Input: part model. Units: mm. Frame: model coordinates. A direction names the side the tool comes from. Give positions to 0.01 mm unless a question says otherwise; leave off trailing zeros. Loops run counter-clockwise (first coordinate to the right, second up) from the corner with the lowest first, then second, coordinate; pieces in that order, holes last. Notation, with made-up numbers: (-36, 64.25) -> (-22, 64.25) arc R25 ccw to (-22, 85.25) -> close; hole circle Ø7 at (-11.5, -5.75). An arc over 180 degrees is marked (long way). Answer as a JSON object with one key per item and string values.
```python
from build123d import *

# Parameters (mm, degrees)
F0_R     = 1.651
F1_DEPTH = 0.8128


with BuildPart() as f1:
    # F0 (on Front) → F1 (new body)
    with BuildSketch(Plane.XZ):
        with BuildLine():
            Line((-6.35, 36.576), (-8.89, 36.576))
            ThreePointArc((-8.89, 36.576), (-11.584077, 35.460077), (-12.7, 32.766))
            Line((-12.7, 32.766), (-12.7, -35.814))
            ThreePointArc((-12.7, -35.814), (-11.584077, -38.508077), (-8.89, -39.624))
            Line((-8.89, -39.624), (8.89, -39.624))
            ThreePointArc((8.89, -39.624), (11.584077, -38.508077), (12.7, -35.814))
            Line((12.7, -35.814), (12.7, 32.766))
            ThreePointArc((12.7, 32.766), (11.584077, 35.460077), (8.89, 36.576))
            Line((8.89, 36.576), (6.35, 36.576))
            Line((6.35, 36.576), (-6.35, 36.576))
        make_face()
        with Locations((-8.098364, -35.367535)):
            Circle(F0_R, mode=Mode.SUBTRACT)
        with Locations((0, -35.367535)):
            Circle(F0_R, mode=Mode.SUBTRACT)
        with Locations((8.098364, -35.367535)):
            Circle(F0_R, mode=Mode.SUBTRACT)
        with BuildLine():
            ThreePointArc((2.921, 4.463106), (0, -5.334), (-2.921, 4.463106))
            Line((-2.921, 4.463106), (-2.921, 10.795))
            ThreePointArc((-2.921, 10.795), (0, 13.716), (2.921, 10.795))
            Line((2.921, 10.795), (2.921, 4.463106))
        make_face(mode=Mode.SUBTRACT)
        with Locations((-8.098364, 32.319535)):
            Circle(F0_R, mode=Mode.SUBTRACT)
        with Locations((0, 32.319535)):
            Circle(F0_R, mode=Mode.SUBTRACT)
        with Locations((8.098364, 32.319535)):
            Circle(F0_R, mode=Mode.SUBTRACT)
        with BuildLine():
            Line((-6.35, 45.466), (-6.35, 36.576))
            Line((-6.35, 36.576), (6.35, 36.576))
            Line((6.35, 36.576), (6.35, 45.466))
            ThreePointArc((6.35, 45.466), (5.234077, 48.160077), (2.54, 49.276))
            Line((2.54, 49.276), (-2.54, 49.276))
            ThreePointArc((-2.54, 49.276), (-5.234077, 48.160077), (-6.35, 45.466))
        make_face()
        with Locations((0, 42.926)):
            Circle(F0_R, mode=Mode.SUBTRACT)
    extrude(amount=F1_DEPTH)


solid = f1.part
```
Q1. Draft query along Z for faces 1 (the cylindrical face through (11.55, -0.4, -38.54)), 2 (the flat face through (-6, 0, 5)), 3 (the cylindrical face through (8.86, -0.401, 30.855)). Return one class per face: +Z half, -Z half, draft (parallel to the pull), parting line (faces both ways), or undercut.
Evaluation:
{"face 1": "-Z half", "face 2": "draft", "face 3": "undercut"}
Q2. Access query for faces 4 (the cylindrical face through (-0.064, -0.401, 13.715)), 5 (the cylindrical face through (-5.204, -0.401, 48.19)). Directions: +Z, -Z, +X, -X, +Y, -Y. A direction counts if a zero-diameter tool reaches every point of the face in a straight line with its end or side. Return the directions, or none.
Evaluation:
{"face 4": "+Y, -Y", "face 5": "+Z, -X, +Y, -Y"}
Q3. Section C-C, the plane y = -0.15. Give the number of separate pieces and of enclosed holes in the cut face, then the cut area to 3 significant figures.
Evaluation:
{"separate pieces": "1", "enclosed holes": "8", "area": "1,880 mm2"}
Q4. Pin query (flat end, axial travel): pin 1 (2.5 mm diameter, centred on x = 0, z = -35.37, fed in from +Y). Return the tip coordinate at first contact, or that it passes through.
Evaluation:
{"pin 1": "passes through"}
Q5. Section B-B, the plane x = 0. Return the cut outline in (y, z) (3 decimals).
Evaluation:
{"outline": "(-0.813, -39.624) -> (0, -39.624) -> (0, -37.019) -> (-0.813, -37.019) -> close; (-0.813, -33.717) -> (0, -33.717) -> (0, -5.334) -> (-0.813, -5.334) -> close; (-0.813, 13.716) -> (0, 13.716) -> (0, 30.669) -> (-0.813, 30.669) -> close; (-0.813, 33.971) -> (0, 33.971) -> (0, 41.275) -> (-0.813, 41.275) -> close; (-0.813, 44.577) -> (0, 44.577) -> (0, 49.276) -> (-0.813, 49.276) -> close"}
Q6. Section D-D, the plane x = 10.5. Return the cut outline in (y, z), then the cut area to 3 significant figures.
Evaluation:
{"outline": "(-0.81, -39.27) -> (0, -39.27) -> (0, 36.22) -> (-0.81, 36.22) -> close", "area": "61.4 mm2"}
Q7. Ray query, line 1 along Z through (x, y) = (0, -0.45) (3 decimals); line 2 along Z through (x, y) = (2, -0.4); line 3 along Z through (x, y) = (-3.75, -0.15). Return the intervals inside material, ascending.
Evaluation:
{"line 1": "z = -39.624 to -37.019, -33.717 to -5.334, 13.716 to 30.669, 33.971 to 41.275, 44.577 to 49.276", "line 2": "z = -39.62 to -4.94, 12.92 to 49.28", "line 3": "z = -39.62 to -3.79, 3.79 to 49.08"}
Q8. Section A-A, the plane z = 0. Return the cut outline in (x, y).
Evaluation:
{"outline": "(-12.7, -0.81) -> (-5.33, -0.81) -> (-5.33, 0) -> (-12.7, 0) -> close; (5.33, -0.81) -> (12.7, -0.81) -> (12.7, 0) -> (5.33, 0) -> close"}
